Design review of the part built by this model. Coordinates are the model's own, in mm. A direction names the side the tool comes from. Give positions to 0.01 mm unless a question says otherwise; leave off trailing zeros. Write each loop counter-clockwise with the first axis right and the second up, starting at its lowest first coordinate (ties: lowest second). Pieces come first, ordered by that corner, then holes.
```python
from build123d import *

# Parameters (mm, degrees)
SKETCH1_W           = 101.6
SKETCH1_H           = 219.075
BOSS_EXTRUDE2_DEPTH = 114.3
SKETCH2_R           = 101.6
CUT_EXTRUDE1_DEPTH  = 219.075
FILLET1_R           = 90
SKETCH3_W           = 35.162695898
SKETCH3_H           = 71.534417327
BOSS_EXTRUDE3_DEPTH = 219.075
CUT_EXTRUDE2_DEPTH  = 219.3
FILLET2_R           = 80
FILLET3_R           = 10
BOSS_EXTRUDE5_DEPTH = 219.075
FILLET5_R           = 100
FILLET7_R           = 100
FILLET11_R          = 100
FILLET12_R          = 100


with BuildPart() as part:
    # Sketch1 → Boss-Extrude2 (new body)
    with BuildSketch(Plane(origin=(0, 0, 0), x_dir=(1, 0, 0), z_dir=(0, 1, 0))):
        Rectangle(SKETCH1_W, SKETCH1_H)
    extrude(amount=BOSS_EXTRUDE2_DEPTH)

    # Sketch2 → Cut-Extrude1 (cut)
    with BuildSketch(Plane.XY.offset(109.5375)):
        with Locations((-73.196036425, 0)):
            Circle(SKETCH2_R)
    extrude(amount=-CUT_EXTRUDE1_DEPTH, mode=Mode.SUBTRACT)

    # Fillet1
    fillet1_edges = [part.edges().sort_by_distance(p)[0] for p in [
        (50.8, 114.3, 0),
    ]]
    fillet(fillet1_edges, radius=FILLET1_R)

    # Sketch3 → Boss-Extrude3 (add)
    with BuildSketch(Plane.XY.offset(109.5375)):
        with Locations((54.990158277, 35.767208663)):
            Rectangle(SKETCH3_W, SKETCH3_H)
    extrude(amount=-BOSS_EXTRUDE3_DEPTH)

    # Sketch4 → Cut-Extrude2 (cut)
    with BuildSketch(Plane.XY.offset(109.5375)):
        with BuildLine():
            Line((37.408810328, 71.534417327), (72.571506226, 71.534417327))
            Line((72.571506226, 71.534417327), (72.571506226, 7.917200167))
            add(Edge.make_bspline(
                [(37.408810328, 71.534417327), (40.159862315, 31.272718553), (72.571506226, 7.917200167)],
                knots=[0, 0, 0, 1, 1, 1], degree=2))
        make_face()
    extrude(amount=-CUT_EXTRUDE2_DEPTH, mode=Mode.SUBTRACT)

    # Fillet2
    fillet2_edges = [part.edges().sort_by_distance(p)[0] for p in [
        (37.408810328, 71.534417327, 0),
    ]]
    fillet(fillet2_edges, radius=FILLET2_R)

    # Fillet3
    fillet3_edges = [part.edges().sort_by_distance(p)[0] for p in [
        (72.571506226, 7.917200167, 0),
    ]]
    fillet(fillet3_edges, radius=FILLET3_R)

    # Sketch5 → Boss-Extrude5 (add)
    with BuildSketch(Plane.XY.offset(109.5375)):
        Polygon((-80.8, 99.100845367), (-80.8, 110.100845367), (-50.8, 114.3), (-50.8, 99.100845367), align=None)
    extrude(amount=-BOSS_EXTRUDE5_DEPTH)

    # Fillet5
    # the kernel refuses this fillet: 100 mm, written as the material it adds along each edge
    with BuildSketch(Plane(origin=(-50.8, 99.100845367, -109.5375), x_dir=(0.6243262651126902, -0.7811636926345457, 0), z_dir=(0, 0, 1))) as fillet5_piece_1:
        with BuildLine():
            CenterArc((65.135381338, -78.674577281), FILLET5_R, 51.882430425, 89.484815402)
            Line((-12.980987926, -16.24195077), (-14.543315311, -14.99329824))
            Line((-14.543315311, -14.99329824), (-1.562327385, 1.24865253))
            Line((-1.562327385, 1.24865253), (-1.24865253, 1.562327385))
            ThreePointArc((-1.24865253, 1.562327385), (63.431548535, 24.233768828), (128.097651386, 1.573491546))
            Line((128.097651386, 1.573491546), (126.863097071, 0))
        make_face()
    extrude(amount=219.075)

    # Fillet7
    fillet7_edges = [part.edges().sort_by_distance(p)[0] for p in [
        (-50.8, 114.3, 0),
    ]]
    fillet(fillet7_edges, radius=FILLET7_R)

    # Fillet11
    # the kernel refuses this fillet: 100 mm, written as the material it takes off along each edge
    with BuildSketch(Plane(origin=(-80.8, -150.899154633, -109.5375), x_dir=(1, 0, 0), z_dir=(0, 1, 0))) as fillet11_piece_1:
        with BuildLine():
            CenterArc((FILLET11_R, -FILLET11_R), FILLET11_R, 90, 90)
            Line((0, -FILLET11_R), (0, 0))
            Line((0, 0), (FILLET11_R, 0))
        make_face()
    extrude(amount=511, mode=Mode.SUBTRACT)

    # Fillet12
    # the kernel refuses this fillet: 100 mm, written as the material it takes off along each edge
    with BuildSketch(Plane(origin=(-80.8, -150.899154633, 109.5375), x_dir=(1, 0, 0), z_dir=(0, 1, 0))) as fillet12_piece_1:
        with BuildLine():
            CenterArc((FILLET12_R, FILLET12_R), FILLET12_R, 180, 90)
            Line((0, FILLET12_R), (0, 0))
            Line((0, 0), (FILLET12_R, 0))
        make_face()
    extrude(amount=511, mode=Mode.SUBTRACT)


solid = part.part
```
(1) Consider section A-A, the plane x = -64.5. Give the boundary of the cut face in (y, z).
Resolved:
outline: (98.85, -64.26) - (112.38, -64.26) - (112.38, 64.26) - (98.85, 64.26) - close
(2) Tool access review of faces 1 (the face through (-66.843, 112.054, 1.029)), 2 (the face through (-75, 99.101, 1)): name each direction out of +Z, -Z, +X, -X, +Y, -Y from which nothing blocks a thin tool from reaching the whole face with its end or side.
Resolved:
face 1: +Z, -Z, -X, +Y
face 2: +Z, -Z, -X, -Y
(3) Clearance check with flat-ended pins moving along their axes: P1, Ø3, axis at y = 36, z = -11.5, coming from the +X side; P2, Ø10, axis at x = -74, z = -17, coming from the -Y side; P3, Ø4, axis at y = 40.5, z = -29, coming from the +X side. State where each tip first meets the part, or that it passes through.
Resolved:
P1: stops at x = 48.14
P2: stops at y = 99.07
P3: stops at x = 46
(4) To check wall thickness, follow L1, parallel to X at y = 89.5, z = 21; L2, parallel to X at y = 68, z = -4.5; L3, parallel to Y at x = -23, z = -75. State the ranges of each line that lie inside material, in increasing order.
Resolved:
L1: x = -28.84 to 20.46
L2: x = 0.88 to 35.2
L3: y = 86.5 to 112.83
